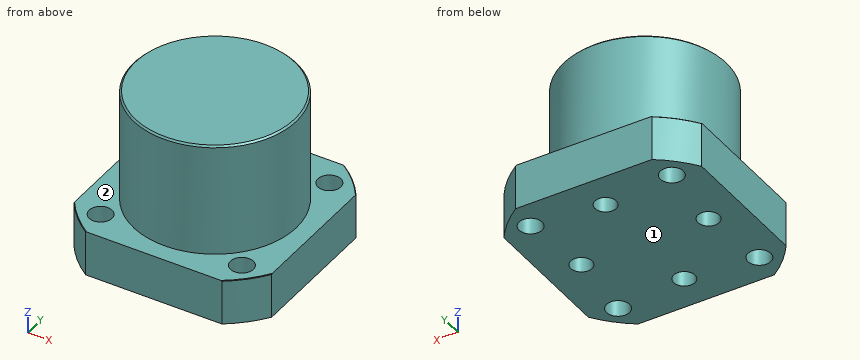
from build123d import *

# Parameters (mm, degrees)
F0_R     = 36.5125
F1_DEPTH = 50.8
F2_R     = 53.975
F3_DEPTH = 20.32
F4_SIZE  = 0.762
F5_SIZE  = 0.254
F6_R     = 69.85
F6_W     = 88.9
F6_H     = 88.9
F7_DEPTH = 25.4
F8_R     = 4.7752
F8_R_2   = 5.1562
F9_DEPTH = 25.4


with BuildPart() as f1:
    # F0 (on Top) → F1 (new body)
    with BuildSketch(Plane.XY):
        Circle(F0_R)
    extrude(amount=-F1_DEPTH)

    # F2 (on face) → F3 (join)
    with BuildSketch(Plane(origin=(0, 0, -50.8), x_dir=(1, 0, 0), z_dir=(0, 0, -1))):
        Circle(F2_R)
    extrude(amount=F3_DEPTH)

    # F4
    f4_edges = [f1.edges().sort_by_distance(p)[0] for p in [
        (-36.5125, 0, 0),
    ]]
    chamfer(f4_edges, length=F4_SIZE)

    # F5
    f5_edges = [f1.edges().sort_by_distance(p)[0] for p in [
        (-53.975, 0, -50.8),
    ]]
    chamfer(f5_edges, length=F5_SIZE)

    # F6 (on face) → F7 (cut)
    with BuildSketch(Plane(origin=(0, 0, -71.12), x_dir=(1, 0, 0), z_dir=(0, 0, -1))):
        Circle(F6_R)
        Rectangle(F6_W, F6_H, mode=Mode.SUBTRACT)
    extrude(amount=-F7_DEPTH, mode=Mode.SUBTRACT)

    # F8 (on face) → F9 (cut)
    with BuildSketch(Plane(origin=(0, 0, -71.12), x_dir=(1, 0, 0), z_dir=(0, 0, -1))):
        with Locations((-28.575, 0)):
            Circle(F8_R)
        with Locations((28.575, 0)):
            Circle(F8_R)
        with Locations((0, 28.575)):
            Circle(F8_R)
        with Locations((0, -28.575)):
            Circle(F8_R)
        with Locations((-31.75, 31.75)):
            Circle(F8_R_2)
        with Locations((31.75, 31.75)):
            Circle(F8_R_2)
        with Locations((31.75, -31.75)):
            Circle(F8_R_2)
        with Locations((-31.75, -31.75)):
            Circle(F8_R_2)
    extrude(amount=-F9_DEPTH, mode=Mode.SUBTRACT)


solid = f1.part
The model under review builds one solid part; all positions refer to its coordinate system, in mm. Face numbers are marked on the shaded views. A direction names the side the tool comes from. Give positions to 0.01 mm unless a question says otherwise; leave off trailing zeros. Write each loop counter-clockwise with the first axis right and the second up, starting at its lowest first coordinate (ties: lowest second). Pieces come first, ordered by that corner, then holes.
1. Wall thickness on L1, parallel to X at y = 0, z = -54.25; L2, parallel to Y at x = 28, z = -51: over which ranges is each line inside the solid? List them lowest first.
2. Add section C-C, the plane z = -6. Write out the cut boundary in (x, y) (1 decimal), plus the area to 3 significant figures.
3. Add section A-A, the plane x = 0. Write out the cut boundary in (y, z), plus the area to 3 significant figures.
4. For P1, Ø5, axis at x = 29, y = 0, coming from the -Z side; P2, Ø6, axis at x = -31.75, y = -31.75, coming from the +Z side; P3, Ø5, axis at y = 27.5, z = -36.5, coming from the +X side; P4, Ø4, axis at x = -19, z = -27.5, coming from the -Y side, all flat-tipped, find the tip position at first contact; note any pin that passes through.
5. Add section B-B, the plane z = -59. Count the separate pieces of the cut face and the enclosed holes in it, plus the area to 3 significant figures.
6. Tool access review of the marked faces 1 and 2: name each direction out of +Z, -Z, +X, -X, +Y, -Y from which nothing blocks a thin tool from reaching the whole face with its end or side.
Worked answers:
1. L1: x = -44.45 to -33.35, -23.8 to 23.8, 33.35 to 44.45
1. L2: y = -44.45 to -35.29, -28.21 to -4.74, 4.74 to 28.21, 35.29 to 44.45
2. outline: circle Ø73 at (0, 0)
2. area: 4,190 mm2
3. outline: (-44.45, -71.12) - (-33.35, -71.12) - (-33.35, -45.72) - (-23.8, -45.72) - (-23.8, -71.12) - (23.8, -71.12) - (23.8, -45.72) - (33.35, -45.72) - (33.35, -71.12) - (44.45, -71.12) - (44.45, -50.8) - (36.51, -50.8) - (36.51, -0.76) - (35.75, 0) - (-35.75, 0) - (-36.51, -0.76) - (-36.51, -50.8) - (-44.45, -50.8) - close
3. area: 5,030 mm2
4. P1: stops at z = -45.72
4. P2: passes through
4. P3: stops at x = 26.61
4. P4: stops at y = -32.31
5. separate pieces: 1
5. enclosed holes: 8
5. area: 6,950 mm2
6. face 1: -Z, +X, -X, +Y, -Y
6. face 2: +Z
